Model file for the job. Use its own axes, mm. A direction names the side the tool comes from. Coordinates: 2 decimals unless noted, no trailing zeros. Order: outer loops, then holes, each group sorted by start corner. A loop starts at its lowest first (then second) coordinate and runs counter-clockwise, first axis right, second up.
from build123d import *

# Parameters (mm, degrees)
EXTRUDE_1_DEPTH     = 160
SHELL_1_T           = -1.5
SKETCH_2_W          = 210
SKETCH_2_H          = 185
CUT_EXTRUDE_1_DEPTH = 200
CHAMFER_1_SIZE      = 13
CHAMFER_1_SIZE2     = 22.516660498
SKETCH_6_W          = 247
SKETCH_6_H          = 80
CUT_EXTRUDE_2_DEPTH = 200
FILLET_1_R          = 10
FILLET_2_R          = 10


with BuildPart() as part:
    # 草图1 → 凸台-拉伸1 (new body)
    with BuildSketch(Plane(origin=(0, 0, 0), x_dir=(1, 0, 0), z_dir=(0, 1, 0))):
        Polygon((-150, 125), (150, 125), (150, -125), (-150, -125), (-300, -110), (-300, 110), align=None)
    extrude(amount=EXTRUDE_1_DEPTH)

    # 抽壳1
    shell_1_openings = [part.faces().sort_by_distance(p)[0] for p in [
        (-71.428571429, 160, 0),
    ]]
    offset(amount=SHELL_1_T, openings=shell_1_openings, kind=Kind.INTERSECTION)

    # 草图2 → 切除-拉伸1 (cut)
    with BuildSketch(Plane.ZY.offset(300)):
        with Locations((0, 107.5)):
            Rectangle(SKETCH_2_W, SKETCH_2_H)
    extrude(amount=-CUT_EXTRUDE_1_DEPTH, mode=Mode.SUBTRACT)

    # 倒角1
    chamfer_1_edges = [part.edges().sort_by_distance(p)[0] for p in [
        (-298.5, 1.5, 0),
    ]]
    chamfer_1_side = [part.faces().sort_by_distance(p)[0] for p in [
        (-298.5, 80.75, 105.953001276),
    ]]
    chamfer(chamfer_1_edges, length=CHAMFER_1_SIZE, length2=CHAMFER_1_SIZE2, reference=chamfer_1_side[0])

    # 草图6 → 切除-拉伸2 (cut)
    with BuildSketch(Plane(origin=(150, 0, 0), x_dir=(0, 0, -1), z_dir=(1, 0, 0))):
        with Locations((0, 120)):
            Rectangle(SKETCH_6_W, SKETCH_6_H)
    extrude(amount=-CUT_EXTRUDE_2_DEPTH, mode=Mode.SUBTRACT)

    # 圆角1
    fillet_1_edges = [part.edges().sort_by_distance(p)[0] for p in [
        (-275.983339502, 1.5, 0),
    ]]
    fillet(fillet_1_edges, radius=FILLET_1_R)

    # 圆角2
    # the kernel refuses this fillet: 10 mm, written as the material it adds along each edge
    with BuildSketch(Plane(origin=(148.5, 1.5, -123.5), x_dir=(0, 0, 1), z_dir=(-1, 0, 0))) as fillet_2_piece_1_section:
        with BuildLine():
            CenterArc((FILLET_2_R, FILLET_2_R), FILLET_2_R, 180, 90)
            Line((0, FILLET_2_R), (0, 0))
            Line((0, 0), (FILLET_2_R, 0))
        make_face()
    fillet_2_piece_1 = extrude(amount=423.425186568, mode=Mode.PRIVATE)
    fillet_2_piece_1 = split(fillet_2_piece_1, bisect_by=Plane(origin=(145.545295182, 1.5, -153.047048175), z_dir=(0.09950371902099917, 0, 0.9950371902099892)), keep=Keep.TOP, mode=Mode.PRIVATE)
    add(fillet_2_piece_1)
    with BuildSketch(Plane(origin=(-274.925186568, 1.5, 123.5), x_dir=(0, 0, -1), z_dir=(1, 0, 0))) as fillet_2_piece_2_section:
        with BuildLine():
            CenterArc((FILLET_2_R, FILLET_2_R), FILLET_2_R, 180, 90)
            Line((0, FILLET_2_R), (0, 0))
            Line((0, 0), (FILLET_2_R, 0))
        make_face()
    fillet_2_piece_2 = extrude(amount=423.425186568, mode=Mode.PRIVATE)
    fillet_2_piece_2 = split(fillet_2_piece_2, bisect_by=Plane(origin=(-273.687562806, 1.5, 111.123762376), z_dir=(0.09950371902099844, 0, -0.9950371902099893)), keep=Keep.TOP, mode=Mode.PRIVATE)
    add(fillet_2_piece_2)


solid = part.part
Q1. Drop flat-ended pins along their axis: P1, Ø4, axis at x = 62.5, z = -33, coming from the -Y side; P2, Ø1.2, axis at x = -299.5, y = 54, coming from the +Z side; P3, Ø1.6, axis at x = 149.5, z = 36.5, coming from the +Y side; P4, Ø6, axis at x = -189.5, y = 32, coming from the -Z side. Give the stop position or say it passes through.
Established:
P1: stops at y = 0
P2: stops at z = 110.11
P3: stops at y = 80
P4: stops at z = -121.35
Q2. Cut at D-D, the plane y = 67. List the corners of the cut face in (x, z).
Established:
outline: (-300, -110) - (-150, -125) - (150, -125) - (150, 125) - (-150, 125) - (-300, 110) - (-300, 105) - (-298.5, 105) - (-298.5, 108.64) - (-149.93, 123.5) - (148.5, 123.5) - (148.5, -123.5) - (-149.93, -123.5) - (-298.5, -108.64) - (-298.5, -105) - (-300, -105) - close
Q3. Probe line 1 (Z direction, x = -124, y = 44); line 2 (X direction, y = 39.5, z = 20.5); line 3 (Y direction, x = -188, z = 19). List the from-to ranges inside material, lowest first.
Established:
line 1: z = -125 to -123.5, 123.5 to 125
line 2: x = 148.5 to 150
line 3: y = 0 to 1.5
Q4. Cut at C-C, the plane z = 12. List the corners of the cut face in (x, y), plus the area to 3 significant figures.
Established:
outline: (-300, 0) - (150, 0) - (150, 80) - (148.5, 80) - (148.5, 1.5) - (-273.3, 1.5) arc R10 cw to (-278.3, 2.84) - (-298.5, 14.5) - (-298.5, 15) - (-300, 15) - close
area: 960 mm2
Q5. Cut at A-A, the plane y = 107. List the corners of the cut face in (x, z), plus the area to 3 significant figures.
Established:
outline: (-300, -110) - (-150, -125) - (150, -125) - (150, -123.5) - (-149.93, -123.5) - (-298.5, -108.64) - (-298.5, -105) - (-300, -105) - close; (-300, 105) - (-298.5, 105) - (-298.5, 108.64) - (-149.93, 123.5) - (150, 123.5) - (150, 125) - (-150, 125) - (-300, 110) - close
area: 1,360 mm2
Q6. Mould opens along Z. For faces 1 (the face through (2, 85, 123.5)), 2 (the face through (-74, 160, -124)), 3 (the face through (2, 79, 125)) say: pulls with the +Z half, pulls with the -Z half, needs draft (parallel to the pull), parting line crosses it, or undercut.
Established:
face 1: undercut
face 2: needs draft
face 3: pulls with the +Z half
Q7. Cut at B-B, the plane x = 50.5. List the corners of the cut face in (y, z).
Established:
outline: (0, -125) - (160, -125) - (160, -123.5) - (11.5, -123.5) arc R10 cw to (1.5, -113.5) - (1.5, 113.5) arc R10 cw to (11.5, 123.5) - (160, 123.5) - (160, 125) - (0, 125) - close
Q8. Which spindle directions (+Z, -Z, +X, -X, +Y, -Y) get a long thin tool onto all of the face, cutting with end or side? Do faces 4 (the face through (-226, 78.9, -117.4)), 5 (the face through (-288.26, 8.59, -1.55)). Say none if no direction does.
Established:
face 4: -Z, -X, +Y, -Y
face 5: +Y
